Geometry check sheet. Reference: the model listing, model coordinates, mm. Face numbers are marked on the shaded views. Round coordinates to 2 decimals unless told otherwise and drop trailing zeros. Write each loop counter-clockwise with the first axis right and the second up, starting at its lowest first coordinate (ties: lowest second). Pieces come first, ordered by that corner, then holes. Notation, with made-up numbers: M 62.25,-32 L 112.25,-32 A18 ccw 112.25,-25 Z; hole C -8.5,81 d6. An arc over 180 degrees is marked long. Answer as CSV lines item,"result". Start each with the question number.
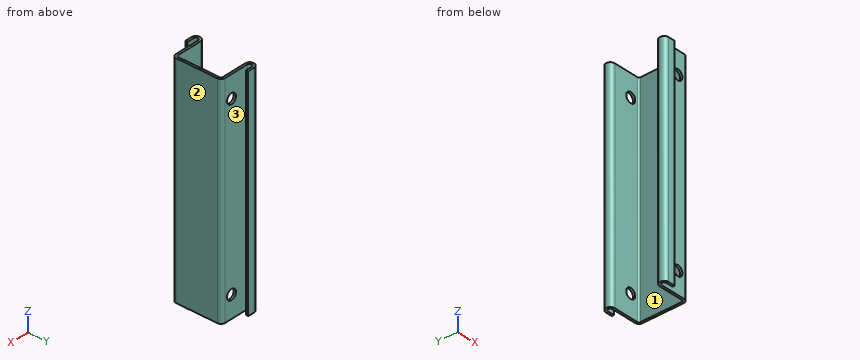
```python
from build123d import *

# Parameters (mm, degrees)
EXTRUDE_1_DEPTH     = 97.4
SKETCH_2_R          = 2.25
CUT_EXTRUDE_1_DEPTH = 97.4


with BuildPart() as part:
    # 草图1 → 凸台-拉伸1 (new body)
    with BuildSketch(Plane.XY):
        with BuildLine():
            Line((-13, 0.7366), (-1.7366, 0.7366))
            ThreePointArc((-1.7366, 0.7366), (-1.215745145, 0.520854855), (-1, 0))
            Line((-1, 0), (-1, -18.5268))
            ThreePointArc((-1, -18.5268), (-1.215745145, -19.047654855), (-1.7366, -19.2634))
            Line((-1.7366, -19.2634), (-13, -19.2634))
            ThreePointArc((-13, -19.2634), (-15, -21.2634), (-13, -23.2634))
            Line((-13, -23.2634), (-10, -23.2634))
            Line((-10, -23.2634), (-10, -22.2634))
            Line((-10, -22.2634), (-13, -22.2634))
            ThreePointArc((-13, -22.2634), (-14, -21.2634), (-13, -20.2634))
            Line((-13, -20.2634), (-1.7366, -20.2634))
            ThreePointArc((-1.7366, -20.2634), (-0.508638364, -19.754761636), (0, -18.5268))
            Line((0, -18.5268), (0, 0))
            ThreePointArc((0, 0), (-0.508638364, 1.227961636), (-1.7366, 1.7366))
            Line((-1.7366, 1.7366), (-13, 1.7366))
            ThreePointArc((-13, 1.7366), (-14, 2.7366), (-13, 3.7366))
            Line((-13, 3.7366), (-10, 3.7366))
            Line((-10, 3.7366), (-10, 4.7366))
            Line((-10, 4.7366), (-13, 4.7366))
            ThreePointArc((-13, 4.7366), (-15, 2.7366), (-13, 0.7366))
        make_face()
    extrude(amount=EXTRUDE_1_DEPTH)

    # 草图2 → 切除-拉伸1 (cut)
    with BuildSketch(Plane.XZ.offset(20.2634)):
        with Locations((-5, 87.65)):
            Circle(SKETCH_2_R)
        with Locations((-5, 9.75)):
            Circle(SKETCH_2_R)
    extrude(amount=-CUT_EXTRUDE_1_DEPTH, mode=Mode.SUBTRACT)


solid = part.part
```
1) Section check A-A, the plane x = -5. Record the cut outline in (y, z), plus the area to 3 significant figures.
2) Scan lines: line 1 (Y direction, x = -13, z = 23); line 2 (Z direction, x = -5, y = 1.3); line 3 (Y direction, x = -8.5, z = 83). Record each from-to range of solid material in increasing order. Write a range as from..to.
3) Section check D-D, the plane z = 52.5. Record the cut outline in (x, y), plus the area to 3 significant figures.
4) Mould release check, pull along Y, two halves, no side actions. Record for the marked faces 1, 2 and 3: released by +Y, released by -Y, zero draft, split by the parting line, or undercut.
5) Section check B-B, the plane z = 9.75. Record the cut outline in (x, y), plus the area to 3 significant figures.
6) Section check C-C, the plane x = -11.5. Record the cut outline in (y, z).
7) Go/stop test with flat-tipped pins: pin 1 (5.5 mm diameter, centred on x = -6, z = 46.5, fed in from -Y); pin 2 (2 mm diameter, centred on y = -16, z = 29, fed in from -X); pin 3 (2 mm diameter, centred on y = -19.5, z = 71.5, fed in from -X). Record where each tip stops, or that it passes through.
Results:
1,outline,"M -20.26,0 L -19.26,0 L -19.26,7.5 L -20.26,7.5 Z; M -20.26,12 L -19.26,12 L -19.26,85.4 L -20.26,85.4 Z; M -20.26,89.9 L -19.26,89.9 L -19.26,97.4 L -20.26,97.4 Z; M 0.74,0 L 1.74,0 L 1.74,7.5 L 0.74,7.5 Z; M 0.74,12 L 1.74,12 L 1.74,85.4 L 0.74,85.4 Z; M 0.74,89.9 L 1.74,89.9 L 1.74,97.4 L 0.74,97.4 Z"
1,area,"177 mm^2"
2,line 1,"y = -23.26..-22.26, -20.26..-19.26, 0.74..1.74, 3.74..4.74"
2,line 2,"z = 0..7.5, 12..85.4, 89.9..97.4"
2,line 3,"y = -20.26..-19.26, 0.74..1.74"
3,outline,"M -13,-23.26 L -10,-23.26 L -10,-22.26 L -13,-22.26 A1 cw -13,-20.26 L -1.74,-20.26 A1.74 ccw 0,-18.53 L 0,0 A1.74 ccw -1.74,1.74 L -13,1.74 A1 cw -13,3.74 L -10,3.74 L -10,4.74 L -13,4.74 A2 ccw -13,0.74 L -1.74,0.74 A0.74 cw -1,0 L -1,-18.53 A0.74 cw -1.74,-19.26 L -13,-19.26 A2 ccw Z"
3,area,"60.4 mm^2"
4,face 1,"undercut"
4,face 2,"zero draft"
4,face 3,"undercut"
5,outline,"M -13,-23.26 L -10,-23.26 L -10,-22.26 L -13,-22.26 A1 cw -13,-20.26 L -7.25,-20.26 L -7.25,-19.26 L -13,-19.26 A2 ccw Z; M -13,0.74 L -7.25,0.74 L -7.25,1.74 L -13,1.74 A1 cw -13,3.74 L -10,3.74 L -10,4.74 L -13,4.74 A2 ccw Z; M -2.75,-20.26 L -1.74,-20.26 A1.74 ccw 0,-18.53 L 0,0 A1.74 ccw -1.74,1.74 L -2.75,1.74 L -2.75,0.74 L -1.74,0.74 A0.74 cw -1,0 L -1,-18.53 A0.74 cw -1.74,-19.26 L -2.75,-19.26 Z"
5,area,"51.4 mm^2"
6,outline,"M -23.26,0 L -22.26,0 L -22.26,97.4 L -23.26,97.4 Z; M -20.26,0 L -19.26,0 L -19.26,97.4 L -20.26,97.4 Z; M 0.74,0 L 1.74,0 L 1.74,97.4 L 0.74,97.4 Z; M 3.74,0 L 4.74,0 L 4.74,97.4 L 3.74,97.4 Z"
7,pin 1,"stops at y = -20.26"
7,pin 2,"stops at x = -1"
7,pin 3,"stops at x = -14.85"
